from build123d import *

# Parameters (mm, degrees)
SKETCH1_W           = 90
SKETCH1_H           = 100
SKETCH1_R           = 2.5
SKETCH1_R_2         = 3.57
BOSS_EXTRUDE1_DEPTH = 3.18
FILLET1_R           = 10
SKETCH2_R           = 2.5
CUT_EXTRUDE1_DEPTH  = 10


with BuildPart() as part:
    # Sketch1 → Boss-Extrude1 (new body)
    with BuildSketch(Plane.XY):
        with Locations((0, -5)):
            Rectangle(SKETCH1_W, SKETCH1_H)
        with Locations((32.3, -42.3)):
            Circle(SKETCH1_R, mode=Mode.SUBTRACT)
        with Locations((-32.3, -42.3)):
            Circle(SKETCH1_R_2, mode=Mode.SUBTRACT)
        with Locations((-32.3, 32.3)):
            Circle(SKETCH1_R_2, mode=Mode.SUBTRACT)
        with Locations((32.3, 32.3)):
            Circle(SKETCH1_R, mode=Mode.SUBTRACT)
    extrude(amount=-BOSS_EXTRUDE1_DEPTH)

    # Fillet1
    fillet1_edges = [part.edges().sort_by_distance(p)[0] for p in [
        (-45, 45, -1.59),
        (45, 45, -1.59),
        (45, -55, -1.59),
        (-45, -55, -1.59),
    ]]
    fillet(fillet1_edges, radius=FILLET1_R)

    # Sketch2 → Cut-Extrude1 (cut)
    with BuildSketch(Plane.XY):
        with Locations((-14.5, -37.5)):
            Circle(SKETCH2_R)
        with Locations((14.5, -37.5)):
            Circle(SKETCH2_R)
        with Locations((-17.523146435, 25.507758855)):
            Circle(SKETCH2_R)
        with Locations((17.523146435, 25.507758855)):
            Circle(SKETCH2_R)
    extrude(amount=-CUT_EXTRUDE1_DEPTH, mode=Mode.SUBTRACT)


solid = part.part
Check sheet for the modelled part. Datum: model origin and axes. Units: mm. Give positions to 0.01 mm unless a question says otherwise; leave off trailing zeros. Loops run counter-clockwise (first coordinate to the right, second up) from the corner with the lowest first, then second, coordinate; pieces in that order, holes last. Notation, with made-up numbers: M 42.5,-29.75 L 85.5,-29.75 A15 cw 85.5,-25.75 Z; hole C 31,89.5 d4. An arc over 180 degrees is marked long. Return JSON: item names as keys, results as strings. Group by question number.
1. Cross-section at C-C on z = -1.4. State how many separate pieces and enclosed holes the cut face has, plus the area to 3 significant figures.
2. Go/stop test with a flat-tipped pin: pin 1 (9.5 mm diameter, centred on x = -32.3, y = -42.3, fed in from +Z). Record where the tip stops, or that it passes through.
3. Thickness scan on L1, parallel to Y at x = -32.3, z = -0.9; L2, parallel to Y at x = 32.3, z = -2.3; L3, parallel to X at y = -44, z = -2.4. Record the ranges inside material, lowest first.
4. Cross-section at D-D on x = -39. Record the boundary of the cut face in (y, z), plus the area to 3 significant figures.
5. Cross-section at A-A on y = -37.5. Record the boundary of the cut face in (x, z).
6. Mould release check, pull along Y, two halves, no side actions. Record for faces 1 (the flat face through (45, -6, -2)), 2 (the cylindrical face through (41.99, 42.15, -1.61)), 3 (the cylindrical face through (15.539, 23.987, -1.568)): released by +Y, released by -Y, zero draft, split by the parting line, or undercut.
7. Cross-section at B-B on x = 33. Record the boundary of the cut face in (y, z), plus the area to 3 significant figures.
Return value:
{
 "1": {"separate pieces": "1", "enclosed holes": "8", "area": "8,720 mm^2"},
 "2": {"pin 1": "z = 0"},
 "3": {"L1": "-55 to -45.87, -38.73 to 28.73, 35.87 to 45", "L2": "-55 to -44.8, -39.8 to 29.8, 34.8 to 45", "L3": "-45 to -35.44, -29.16 to 30.47, 34.13 to 45"},
 "4": {"outline": "M -54.17,-3.18 L 44.17,-3.18 L 44.17,0 L -54.17,0 Z", "area": "313 mm^2"},
 "5": {"outline": "M -45,-3.18 L -17,-3.18 L -17,0 L -45,0 Z; M -12,-3.18 L 12,-3.18 L 12,0 L -12,0 Z; M 17,-3.18 L 45,-3.18 L 45,0 L 17,0 Z"},
 "6": {"face 1": "zero draft", "face 2": "released by +Y", "face 3": "undercut"},
 "7": {"outline": "M -55,-3.18 L -44.7,-3.18 L -44.7,0 L -55,0 Z; M -39.9,-3.18 L 29.9,-3.18 L 29.9,0 L -39.9,0 Z; M 34.7,-3.18 L 45,-3.18 L 45,0 L 34.7,0 Z", "area": "287 mm^2"}
}
